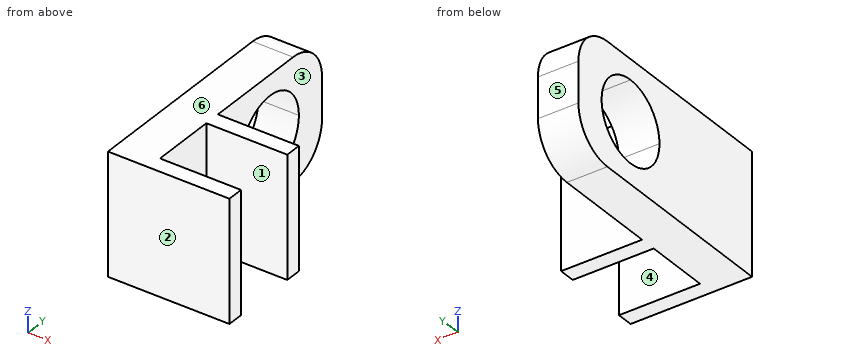
from build123d import *

# Parameters (mm, degrees)
F0_W     = 10
F0_H     = 2
F1_DEPTH = 15
F3_DEPTH = 5
F4_R     = 5


with BuildPart() as f1:
    # F0 (on Top) → F1 (new body)
    with BuildSketch(Plane.XY):
        with Locations((10, 1)):
            Rectangle(F0_W, F0_H)
        with Locations((10, 11)):
            Rectangle(F0_W, F0_H)
        Polygon((0, 30), (0, 0), (5, 0), (5, 2), (5, 10), (5, 12), (5, 30), align=None)
    extrude(amount=F1_DEPTH)

    # F2 (on face) → F3 (cut, through all)
    with BuildSketch(Plane.YZ.offset(5)):
        with BuildLine():
            Line((21, 7.5), (21, 12.5))
            ThreePointArc((21, 12.5), (17.464466, 11.035534), (16, 7.5))
            Line((16, 7.5), (21, 7.5))
        make_face()
        with BuildLine():
            ThreePointArc((21, 2.5), (24.535534, 3.964466), (26, 7.5))
            Line((26, 7.5), (21, 7.5))
            Line((21, 7.5), (21, 2.5))
        make_face()
        with BuildLine():
            ThreePointArc((16, 7.5), (17.464466, 3.964466), (21, 2.5))
            Line((21, 2.5), (21, 7.5))
            Line((21, 7.5), (16, 7.5))
        make_face()
        with BuildLine():
            Line((21, 7.5), (26, 7.5))
            ThreePointArc((26, 7.5), (24.535534, 11.035534), (21, 12.5))
            Line((21, 12.5), (21, 7.5))
        make_face()
    extrude(amount=-F3_DEPTH, mode=Mode.SUBTRACT)

    # F4
    f4_edges = [f1.edges().sort_by_distance(p)[0] for p in [
        (2.5, 30, 15),
        (2.5, 30, 0),
    ]]
    fillet(f4_edges, radius=F4_R)


solid = f1.part
Check sheet for the modelled part. Datum: model origin and axes. Units: mm. Face numbers are marked on the shaded views. A direction names the side the tool comes from. Coordinates: 2 decimals unless noted, no trailing zeros. Write each loop counter-clockwise with the first axis right and the second up, starting at its lowest first coordinate (ties: lowest second). Pieces come first, ordered by that corner, then holes.
Item 1: Cross-section at B-B on x = 12.5. Record the boundary of the cut face in (y, z).
Numbers:
outline: (0, 0) - (2, 0) - (2, 15) - (0, 15) - close; (10, 0) - (12, 0) - (12, 15) - (10, 15) - close
Item 2: Depth check by flat-ended pin: pin 1 Ø1 at (x, z) = (9.5, 7) entering from +Y; pin 2 Ø7.5 at (y, z) = (19, 4.5) entering from +X. Enter the tip coordinate at first touch or a pass-through.
Numbers:
pin 1: stops at y = 12
pin 2: stops at x = 5
Item 3: Mould release check, pull along Y, two halves, no side actions. Record for the marked faces 4, 5 and 6: released by +Y, released by -Y, zero draft, split by the parting line, or undercut.
Numbers:
face 4: undercut
face 5: released by +Y
face 6: zero draft
Item 4: Cross-section at A-A on x = 1.5. Record the boundary of the cut face in (y, z).
Numbers:
outline: (0, 0) - (25, 0) arc R5 ccw to (30, 5) - (30, 10) arc R5 ccw to (25, 15) - (0, 15) - close; hole circle Ø10 at (21, 7.5)
Item 5: Access from +Z, -Z, +X, -X, +Y, -Y to the whole of each face (thin tool, end or side, straight path). Record for the marked faces 1, 2 and 3.
Numbers:
face 1: +Z, -Z, +X
face 2: +Z, -Z, +X, -X, -Y
face 3: +Z, -Z, +X, +Y
Item 6: Cross-section at C-C on z = 8.25. Record the boundary of the cut face in (x, y), then the cut area to 3 significant figures.
Numbers:
outline: (0, 0) - (15, 0) - (15, 2) - (5, 2) - (5, 10) - (15, 10) - (15, 12) - (5, 12) - (5, 16.06) - (0, 16.06) - close; (0, 25.94) - (5, 25.94) - (5, 30) - (0, 30) - close
area: 141 mm2
Item 7: Scan lines: probe 1 along Y at (x, z) = (8, 2.75); probe 2 along Z at (x, y) = (4.25, 21.25); probe 3 along Y at (x, z) = (1.25, 7.75). Record each from-to range of solid material in increasing order.
Numbers:
probe 1: y = 0 to 2, 10 to 12
probe 2: z = 0 to 2.51, 12.49 to 15
probe 3: y = 0 to 16.01, 25.99 to 30
Item 8: Cross-section at D-D on y = 23.75. Record the boundary of the cut face in (x, z).
Numbers:
outline: (0, 0) - (5, 0) - (5, 3.32) - (0, 3.32) - close; (0, 11.68) - (5, 11.68) - (5, 15) - (0, 15) - close
